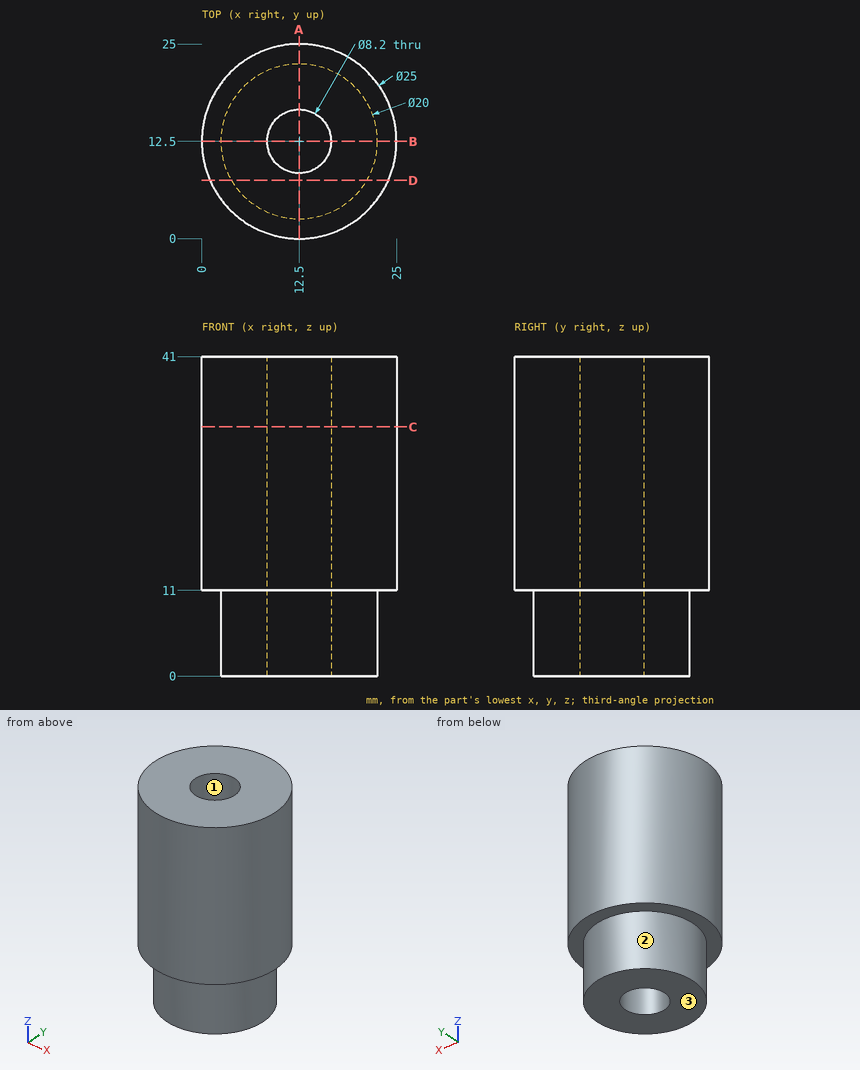
Job drawing, mm, ordinate dimensions from the low corner. One solid piece. Coordinates: 2 decimals unless noted, no trailing zeros. Write each loop counter-clockwise with the first axis right and the second up, starting at its lowest first coordinate (ties: lowest second). Pieces come first, ordered by that corner, then holes. Notation, with made-up numbers: (28, 19) - (47, 19) arc R31 cw to (47, 49) - close; hole circle Ø1 at (47.25, 35). An arc over 180 degrees is marked (long way). Use a Markdown table: item, result. Add a question column.
Item 1: Band-saw the part on A-A, the plane x = 12.5. Give the cut face in (y, z), and give its area (3 significant figures).
Item 2: Band-saw the part on D-D, the plane y = 7.5. Give the cut face in (x, z), and give its area (3 significant figures).
Item 3: Mould opens along Y. For the marked faces 1, 2 and 3 say: pulls with the +Y half, pulls with the -Y half, needs draft (parallel to the pull), parting line crosses it, or undercut.
Item 4: Band-saw the part on C-C, the plane z = 32. Give the cut face in (x, y), and give its area (3 significant figures).
Item 5: Drill centre lines: L1, parallel to X at y = 12.75, z = 22; L2, parallel to Y at x = 12.5, z = 26.5; L3, parallel to Y at x = 12.5, z = 10.5. Where is each one in solid material? Low to high. Write a range as from..to.
Item 6: Flat gauge pins, fed straight in: pin 1 (1.5 mm diameter, centred on x = 10, z = 6, fed in from +Y); pin 2 (1 mm diameter, centred on x = 16, z = 26.5, fed in from -Y); pin 3 (8 mm diameter, centred on y = 4.5, z = 17, fed in from -X). Where does each tip first touch, or does it go through?
Numbers:
| question | item | result |
|---|---|---|
| 1 | outline | (0, 11) - (2.5, 11) - (2.5, 0) - (8.4, 0) - (8.4, 41) - (0, 41) - close; (16.6, 0) - (22.5, 0) - (22.5, 11) - (25, 11) - (25, 41) - (16.6, 41) - close |
| 1 | area | 634 mm2 |
| 2 | outline | (1.04, 11) - (3.84, 11) - (3.84, 0) - (21.16, 0) - (21.16, 11) - (23.96, 11) - (23.96, 41) - (1.04, 41) - close |
| 2 | area | 878 mm2 |
| 3 | face 1 | undercut |
| 3 | face 2 | parting line crosses it |
| 3 | face 3 | needs draft |
| 4 | outline | circle Ø25 at (12.5, 12.5); hole circle Ø8.2 at (12.5, 12.5) |
| 4 | area | 438 mm2 |
| 5 | L1 | 0..8.41, 16.59..25 |
| 5 | L2 | 0..8.4, 16.6..25 |
| 5 | L3 | 2.5..8.4, 16.6..22.5 |
| 6 | pin 1 | y = 22.35 |
| 6 | pin 2 | y = 0.37 |
| 6 | pin 3 | x = 0.66 |
